The model under review builds one solid part; all positions refer to its coordinate system, in mm. A direction names the side the tool comes from. Round coordinates to 2 decimals unless told otherwise and drop trailing zeros. Write each loop counter-clockwise with the first axis right and the second up, starting at its lowest first coordinate (ties: lowest second). Pieces come first, ordered by that corner, then holes. Notation, with made-up numbers: (6.5, -20.5) - (35.5, -20.5) arc R14 cw to (35.5, 6.5) - close; hole circle Ø8 at (10, 55.25). An arc over 180 degrees is marked (long way). Return JSON: item names as keys, results as strings.
Autodesk Inventor part; units mm, degrees
ref_plane "YZ Plane" through (0, 0, 0) normal (1, 0, 0) x (0, 1, 0)
ref_plane "XZ Plane" through (0, 0, 0) normal (0, 1, 0) x (-1, 0, 0)
ref_plane "XY Plane" through (0, 0, 0) normal (0, 0, 1) x (1, 0, 0)
sketch "Sketch1" plane through (0, 0, 0) normal (0, 0, 1) x (1, 0, 0)
  line L0 (0, 0) -> (133.35, 0)
  line L1 (133.35, 0) -> (133.35, 50.8)
  line L2 (0, 50.8) -> (0, 0)
  line L3 (0, 50.8) -> (6.35, 50.8)
  line L4 (6.35, 50.8) -> (6.35, 6.35)
  line L5 (6.35, 6.35) -> (127, 6.35)
  line L6 (127, 6.35) -> (127, 50.8)
  line L7 (127, 50.8) -> (133.35, 50.8)
  dimension "d1" = 50.8
  dimension "d2" = 6.35
  dimension "d3" = 44.45
  dimension "d4" = 120.65
  dimension "d5" = 133.35
extrude "Extrusion1" add sketch "Sketch1" along normal blind 6.35
fillet "Fillet1" radius 3.175 2 edges at (66.675, 0, 6.35) (66.675, 0, 0)
sketch "Sketch2" plane through (0, 50.8, 0) normal (0, 1, 0) x (1, 0, 0)
  line L0 (6.35, -6.35) -> (16.515747, 6.26204)
  line L1 (-2.903527, -17.830303) -> (6.35, -6.35)
  line L2 (16.515747, 6.26204) -> (9.563953, 11.86543)
  line L3 (9.563953, 11.86543) -> (-9.855321, -12.226913)
  line L4 (-9.855321, -12.226913) -> (-2.903527, -17.830303)
  line L5 (127, 0) -> (127, -6.35)
  line L6 (127, -6.35) -> (143.198942, -6.35) construction
  line L7 (116.834265, 6.26204) -> (123.786067, 11.86543)
  line L8 (123.786067, 11.86543) -> (143.205318, -12.226913)
  line L9 (143.205318, -12.226913) -> (136.253516, -17.830303)
  line L10 (133.35, -6.35) -> (127, -6.35)
  line L11 (116.834265, 6.26204) -> (136.253516, -17.830303)
  point P0 (0, 0)
extrude "Extrusion2" add sketch "Sketch2" along normal blind 6.35
sketch "Sketch4" plane through (16.515747, 50.8, -6.26204) normal (0.7785715, 0, 0.6275559) x (0.6275559, 0, -0.7785715)
  point P0 (-15.240001, -50.8)
sketch "Sketch5" plane through (16.515747, 50.8, -6.26204) normal (0.7785715, 0, 0.6275559) x (0.6275559, 0, -0.7785715)
  point P0 (-15.240001, -50.8)
sketch "Sketch6" plane through (16.515747, 50.8, -6.26204) normal (0.7785715, 0, 0.6275559) x (0.6275559, 0, -0.7785715)
  line L0 (-30.944292, 6.35) -> (0, 6.35)
  line L1 (-30.944292, 0) -> (-30.944292, 6.35)
  line L2 (-30.944292, 6.35) -> (-30.944292, 0)
  line L3 (0, 0) -> (0, 6.35)
  line L4 (-30.944292, 0) -> (0, 0)
  line L5 (0, 0) -> (0, 6.35)
  line L6 (0, 6.35) -> (-30.944292, 6.35)
  point P0 (-15.240001, -50.8)
extrude "Extrusion3" add sketch "Sketch6" along normal blind 1.5875
sketch "Sketch7" plane through (-9.855321, 50.8, 12.226913) normal (-0.7785715, 0, -0.6275559) x (-0.6275559, 0, 0.7785715)
  line L0 (-30.944292, 6.35) -> (0, 6.35)
  line L1 (0, 0) -> (-30.944292, 0)
  line L2 (-30.944292, 6.35) -> (-30.944292, 0)
  line L3 (-30.944292, 0) -> (0, 0)
  line L4 (0, 6.35) -> (0, 0)
  line L5 (0, 0) -> (0, 6.35)
  line L6 (0, 6.35) -> (-30.944292, 6.35)
  point P0 (-15.704291, -50.8)
extrude "Extrusion4" add sketch "Sketch7" along normal blind 1.5875
sketch "Sketch8" plane through (136.253516, 50.8, 17.830303) normal (-0.7785718, 0, 0.6275555) x (0.6275555, 0, 0.7785718)
  line L0 (-30.944277, 6.35) -> (0, 6.35)
  line L1 (0, 0) -> (0, 6.35)
  line L2 (-30.944277, 6.35) -> (0, 6.35)
  line L3 (0, 6.35) -> (0, 0)
  line L4 (0, 0) -> (-30.944277, 0)
  line L5 (-30.944277, 0) -> (-30.944277, 6.35)
  line L6 (-30.944277, 0) -> (-30.944277, 6.35)
  point P0 (-99.388813, -50.8)
extrude "Extrusion5" add sketch "Sketch8" along normal blind 1.5875
sketch "Sketch9" plane through (123.786067, 50.8, -11.86543) normal (0.7785718, 0, -0.6275555) x (-0.6275555, 0, -0.7785718)
  line L0 (-30.944277, 6.35) -> (0, 6.35)
  line L1 (-30.944277, 6.35) -> (0, 6.35)
  line L2 (0, 0) -> (-30.944277, 0)
  line L3 (0, 6.35) -> (0, 0)
  line L4 (0, 0) -> (-30.944277, 0)
  line L5 (-30.944277, 0) -> (-30.944277, 6.35)
  point P0 (68.444536, -50.8)
extrude "Extrusion6" add sketch "Sketch9" along normal blind 1.5875
sketch "Sketch10" plane through (125.02205, 50.8, -12.861674) normal (0.7785718, 0, -0.6275555) x (-0.6275555, 0, -0.7785718)
  point P0 (68.444536, -50.8)
sketch "Sketch11" plane through (125.02205, 50.8, -12.861674) normal (0.7785718, 0, -0.6275555) x (-0.6275555, 0, -0.7785718)
  line L0 (0, 0) -> (0, 6.35)
  line L1 (0, 0) -> (0, 12.7)
  line L2 (-30.944277, 6.35) -> (-30.944277, 0)
  line L3 (0, 0) -> (-30.944277, 0)
  line L4 (-30.944277, 0) -> (-30.944277, 12.7)
  line L5 (-30.944277, 12.7) -> (0, 12.7)
  point P0 (68.444536, -50.8)
  point P1 (0, 6.35)
  point P2 (-30.944277, 6.35)
  dimension "d40" = 12.7
extrude "Extrusion7" add sketch "Sketch11" along normal blind 3.175
sketch "Sketch12" plane through (135.017533, 50.8, 18.826547) normal (-0.7785718, 0, 0.6275555) x (0.6275555, 0, 0.7785718)
  line L0 (0, 12.7) -> (0, 0)
  line L1 (0, 0) -> (0, 12.7)
  line L2 (-30.944277, 12.7) -> (0, 12.7)
  line L3 (0, 12.7) -> (-30.944277, 12.7)
  line L4 (0, 0) -> (-30.944277, 0)
  line L5 (-30.944277, 12.7) -> (-30.944277, 0)
  line L6 (-30.944277, 0) -> (0, 0)
  point P0 (-99.388813, -50.8)
extrude "Extrusion8" add sketch "Sketch12" along normal blind 3.175
sketch "Sketch13" plane through (-11.091303, 50.8, 11.230668) normal (-0.7785715, 0, -0.6275559) x (-0.6275559, 0, 0.7785715)
  line L0 (-30.944292, 0) -> (-30.944292, 6.35)
  line L1 (-30.944292, 0) -> (-30.944292, 12.7)
  line L2 (0, 6.35) -> (0, 0)
  line L3 (-30.944292, 0) -> (0, 0)
  line L4 (0, 0) -> (0, 12.7)
  line L5 (0, 12.7) -> (-30.944292, 12.7)
  point P0 (-15.704291, -50.8)
  point P1 (-30.944292, 6.35)
  dimension "d45" = 12.7
extrude "Extrusion9" add sketch "Sketch13" along normal blind 3.175
sketch "Sketch14" plane through (17.751729, 50.8, -5.265795) normal (0.7785715, 0, 0.6275559) x (0.6275559, 0, -0.7785715)
  line L0 (-30.944292, 0) -> (-30.944292, 6.35)
  line L1 (-30.944292, 0) -> (-30.944292, 12.7)
  line L2 (-30.944292, 12.7) -> (0, 12.7)
  line L3 (-30.944292, 12.7) -> (0, 12.7)
  line L4 (0, 0) -> (0, 6.35)
  line L5 (0, 12.7) -> (0, 0)
  line L6 (0, 0) -> (-30.944292, 0)
  point P0 (-15.240001, -50.8)
  point P1 (0, 6.35)
  point P2 (-30.944292, 12.7)
  point P3 (-30.944292, 6.35)
  dimension "d8" = 3.175
extrude "Extrusion10" add sketch "Sketch14" along normal blind 3.175
fillet "Fillet4" radius 6.35 8 edges at (133.35, 50.8, 3.175) (130.175, 50.8, 0) (127, 50.8, 3.175) (130.175, 50.8, 6.35) (6.35, 50.8, 3.175) (3.175, 50.8, 6.35) (0, 50.8, 3.175) (3.175, 50.8, 0)
properties part number "landing_3DPrint"
(1) Add section D-D (y = 33.5). Write out the cut boundary in (x, z).
Filled in:
{"outline": "(0, 0) - (6.35, 0) - (6.35, 6.35) - (0, 6.35) - close; (127, 0) - (133.35, 0) - (133.35, 6.35) - (127, 6.35) - close"}
(2) Add section A-A (y = 52.5). Write out the cut boundary in (x, z).
Filled in:
{"outline": "(-13.56, 9.24) - (5.86, -14.85) - (20.22, -3.27) - (0.8, 20.82) - close; (113.13, -3.27) - (127.49, -14.85) - (146.91, 9.24) - (132.55, 20.82) - close"}
(3) Wall thickness on line 1 (X direction, y = 40.5, z = 1.5); line 2 (X direction, y = 59.5, z = -1.5); line 3 (Y direction, x = 116.5, z = -5.5): over which ranges is each line inside the solid? List them lowest first.
Filled in:
{"line 1": "x = 0 to 6.35, 127 to 133.35", "line 2": "x = -4.91 to -0.83, 14.72 to 18.79, 114.56 to 118.63, 134.18 to 138.26", "line 3": "y = 50.8 to 57.15"}
(4) For faces 1 (the flat face through (120.21, 55.65, -8.983)), 2 (the flat face through (134.868, 60.369, -0.647)), 3 (the cylindrical face through (9, 49.61, 3.37)), list the 3-axis set-ups (+Z, -Z, +X, -X, +Y, -Y) from which the entire face can be reached by the end or side of a thin tool; tool diameter is ignored.
Filled in:
{"face 1": "-Z, +Y, -Y", "face 2": "+Y", "face 3": "+Z, -Z"}
(5) Mouldability with a two-part tool opening along Z and no side actions: class faces 4 (the flat face through (66, 6.35, 3)), 5 (the flat face through (4, 57.15, 3)), 6 (the flat face through (122.7, 56.689, 8.604)) as released by +Z, released by -Z, zero draft, split by the parting line, or undercut.
Filled in:
{"face 4": "zero draft", "face 5": "undercut", "face 6": "released by +Z"}
(6) Add section B-B (z = -11). Write out the cut boundary in (x, y), plus the area to 3 significant figures.
Filled in:
{"outline": "(2.75, 50.8) - (10.64, 50.8) - (10.64, 57.15) - (6.83, 57.15) - (6.83, 63.5) - (2.75, 63.5) - close; (122.71, 50.8) - (130.6, 50.8) - (130.6, 63.5) - (126.52, 63.5) - (126.52, 57.15) - (122.71, 57.15) - close", "area": "152 mm2"}
(7) Clearance check with flat-ended pins moving along their axes: pin 1 Ø2 at (x, z) = (107, 3.5) entering from +Y; pin 2 Ø3 at (x, z) = (54, 1.5) entering from -Y; pin 3 Ø10 at (y, z) = (46.5, 15.5) entering from +X. State where each tip first meets the part, or that it passes through.
Filled in:
{"pin 1": "stops at y = 6.35", "pin 2": "stops at y = 0", "pin 3": "stops at x = 142.31"}
